from build123d import *

# Parameters (mm, degrees)
F2_DEPTH  = 25.4
F3_DEPTH  = 25.4
F5_DEPTH  = 12.7
F7_DEPTH  = 12.7
F9_DEPTH  = 25.4
F10_DEPTH = 12.7
F11_DEPTH = 12.7


with BuildPart() as f2:
    # F1 (on Right) → F2 (new body)
    with BuildSketch(Plane.YZ):
        Polygon((0, 6.35), (0, 0), (38.1, 0), (38.1, 6.35), (25.4, 6.35), (12.7, 6.35), align=None)
        Polygon((25.4, 6.35), (38.1, 6.35), (38.1, 25.4), (25.4, 25.4), (25.4, 19.05), (12.7, 19.05), (12.7, 12.7), (25.4, 12.7), align=None)
    extrude(amount=F2_DEPTH)

    # F0 (on Front) → F3 (join)
    with BuildSketch(Plane.XZ):
        Polygon((0, 6.35), (0, 0), (25.4, 0), (25.4, 6.35), (19.05, 6.35), align=None)
        Polygon((0, 19.05), (0, 6.35), (19.05, 6.35), (19.05, 11.1125), (8.4666666667, 19.05), align=None)
        Polygon((19.05, 6.35), (25.4, 6.35), (19.05, 11.1125), align=None)
        Polygon((0, 25.4), (0, 19.05), (8.4666666667, 19.05), align=None)
    extrude(amount=-F3_DEPTH)

    # F4 (on face) → F5 (cut)
    with BuildSketch(Plane.XZ):
        Polygon((25.4, 6.35), (0, 25.4), (0, 6.35), align=None)
    extrude(amount=-F5_DEPTH, mode=Mode.SUBTRACT)

    # F7 (cut): a face of the model
    f7_faces = [f2.faces().sort_by_distance(p)[0] for p in [
        (14.6755555556, 25.4, 22.4366666667),
    ]]
    extrude(f7_faces, amount=-F7_DEPTH, mode=Mode.SUBTRACT)

    # F8 (on face) → F9 (cut)
    with BuildSketch(Plane.XZ.offset(-12.7)):
        Polygon((8.4666666667, 19.05), (8.3384562082, 19.05), (17.2284582002, 12.7), (25.4, 12.7), (25.4, 19.05), align=None)
    extrude(amount=-F9_DEPTH, mode=Mode.SUBTRACT)

    # F6 (on face) → F10 (cut)
    with BuildSketch(Plane.XZ.offset(-12.7)):
        Polygon((0, 19.05), (8.4666666667, 19.05), (0, 25.4), align=None)
    extrude(amount=-F10_DEPTH, mode=Mode.SUBTRACT)

    # F11 (cut): a face of the model
    f11_faces = [f2.faces().sort_by_distance(p)[0] for p in [
        (22.5777777778, 25.4, 10.5833333333),
    ]]
    extrude(f11_faces, amount=-F11_DEPTH, mode=Mode.SUBTRACT)


solid = f2.part
The model under review builds one solid part; all positions refer to its coordinate system, in mm. A direction names the side the tool comes from. Round coordinates to 2 decimals unless told otherwise and drop trailing zeros. Loops run counter-clockwise (first coordinate to the right, second up) from the corner with the lowest first, then second, coordinate; pieces in that order, holes last. Notation, with made-up numbers: (-14, -33) -> (44, -33) arc R19 cw to (44, -17) -> close; hole circle Ø9 at (-37, 60). An arc over 180 degrees is marked (long way). Answer as CSV lines item,"result".
1) Tool access review of faces 1 (the face through (2, 25.4, 21)), 2 (the face through (13, 0, 3)): name each direction out of +Z, -Z, +X, -X, +Y, -Y from which nothing blocks a thin tool from reaching the whole face with its end or side.
Geometry results:
face 1,"+Z, +X, -X, -Y"
face 2,"+Z, -Z, +X, -X, -Y"
2) Add section C-C on x = 4. Write out the cut boundary in (y, z), plus the area to 3 significant figures.
Geometry results:
outline,"(0, 0) -> (38.1, 0) -> (38.1, 22.4) -> (25.4, 22.4) -> (25.4, 19.05) -> (12.7, 19.05) -> (12.7, 6.35) -> (0, 6.35) -> close"
area,"607 mm²"
3) Add section B-B on x = 7. Write out the cut boundary in (y, z), plus the area to 3 significant figures.
Geometry results:
outline,"(0, 0) -> (38.1, 0) -> (38.1, 20.15) -> (25.4, 20.15) -> (25.4, 19.05) -> (12.7, 19.05) -> (12.7, 6.35) -> (0, 6.35) -> close"
area,"578 mm²"
4) For P1, Ø6, axis at y = 25.5, z = 15, coming from the +X side; P2, Ø6, axis at y = 14.5, z = 11.5, coming from the -X side; P3, Ø4, axis at x = 17, z = 11, coming from the -Y side; P4, Ø3, axis at x = 9.5, y = 26, coming from the +Z side, all flat-tipped, find the tip position at first contact; note any pin that passes through.
Geometry results:
P1,"stops at x = 17.87"
P2,"stops at x = 0"
P3,"stops at y = 12.7"
P4,"stops at z = 19.4"
5) To check wall thickness, follow line 1 along Y through (x, z) = (2.5, 11.5); line 2 along Z through (x, y) = (15.25, 3.5); line 3 along Z through (x, y) = (3, 18.5). State the ranges of each line that lie inside material, in increasing order. Write a range as from..to.
Geometry results:
line 1,"y = 12.7..38.1"
line 2,"z = 0..6.35"
line 3,"z = 0..19.05"
6) Add section D-D on z = 16.5. Write out the cut boundary in (x, y), plus the area to 3 significant figures.
Geometry results:
outline,"(0, 12.7) -> (11.91, 12.7) -> (11.91, 38.1) -> (0, 38.1) -> close"
area,"302 mm²"
7) Add section A-A on y = 34.5. Write out the cut boundary in (x, z), plus the area to 3 significant figures.
Geometry results:
outline,"(0, 0) -> (25.4, 0) -> (25.4, 6.35) -> (16.93, 12.7) -> (17.23, 12.7) -> (8.34, 19.05) -> (8.47, 19.05) -> (0, 25.4) -> close"
area,"404 mm²"
